For this review, take the finished solid that the model builds, in its own axes (mm). A direction names the side the tool comes from. Coordinates: 2 decimals unless noted, no trailing zeros. Loops run counter-clockwise (first coordinate to the right, second up) from the corner with the lowest first, then second, coordinate; pieces in that order, holes last. Notation, with made-up numbers: (56, -4) -> (101, -4) arc R16 ccw to (101, 20) -> close; hole circle Ø8 at (3.5, -3). An arc over 180 degrees is marked (long way). Answer in a Markdown table with one row per item.
from build123d import *

# Parameters (mm, degrees)
SKETCH1_R                = 2.75
BOSS_EXTRUDE1_DEPTH      = 1
BOSS_EXTRUDE1_DEPTH_BACK = 8.525
CHAMFER1_SIZE            = 10
CHAMFER2_SIZE            = 1
SKETCH2_R                = 1.7
CUT_EXTRUDE1_DEPTH       = 97.192388155
SKETCH3_R                = 1.1
CUT_EXTRUDE2_DEPTH       = 97.192388155
SKETCH4_R                = 3.175
CUT_EXTRUDE3_DEPTH       = 3


with BuildPart() as part:
    # Sketch1 → Boss-Extrude1 (new body, two sides)
    with BuildSketch(Plane.XY) as boss_extrude1_sk:
        Polygon((-1071, 209.41125497), (-1071, 239.41125497), (-1159.192388155, 239.41125497), (-1159.192388155, 259.41125497), (-1167.192388155, 259.41125497), (-1167.192388155, 209.41125497), align=None)
        with Locations((-1122.192388155, 224.41125497)):
            Circle(SKETCH1_R, mode=Mode.SUBTRACT)
        with Locations((-1142.192388155, 224.41125497)):
            Circle(SKETCH1_R, mode=Mode.SUBTRACT)
    extrude(amount=BOSS_EXTRUDE1_DEPTH)
    extrude(boss_extrude1_sk.sketch, amount=-BOSS_EXTRUDE1_DEPTH_BACK)

    # Chamfer1
    chamfer1_edges = [part.edges().sort_by_distance(p)[0] for p in [
        (-1071, 209.41125497, -3.7625),
    ]]
    chamfer(chamfer1_edges, length=CHAMFER1_SIZE)

    # Chamfer2
    chamfer2_edges = [part.edges().sort_by_distance(p)[0] for p in [
        (-1167.192388155, 209.41125497, -3.7625),
        (-1071, 239.41125497, -3.7625),
    ]]
    chamfer(chamfer2_edges, length=CHAMFER2_SIZE)

    # Sketch2 → Cut-Extrude1 (cut, through all)
    with BuildSketch(Plane.ZY.offset(1167.192388155)):
        with Locations((-3.762499999, 249.41125497)):
            Circle(SKETCH2_R)
    extrude(amount=-CUT_EXTRUDE1_DEPTH, mode=Mode.SUBTRACT)

    # Sketch3 → Cut-Extrude2 (cut, through all)
    with BuildSketch(Plane.ZY.offset(1167.192388155)):
        with Locations((-3.762499999, 255.41125497)):
            Circle(SKETCH3_R)
        with Locations((-3.762499999, 243.41125497)):
            Circle(SKETCH3_R)
    extrude(amount=-CUT_EXTRUDE2_DEPTH, mode=Mode.SUBTRACT)

    # Sketch4 → Cut-Extrude3 (cut)
    with BuildSketch(Plane.ZY.offset(1167.192388155)):
        with Locations((-3.762499999, 249.41125497)):
            Circle(SKETCH4_R)
    extrude(amount=-CUT_EXTRUDE3_DEPTH, mode=Mode.SUBTRACT)


solid = part.part
Item 1: Take a section at D-D, the plane x = -1124. State the section outline as (y, z) points (3 decimals), and give its area (3 significant figures).
Worked answers:
| item | result |
|---|---|
| outline | (209.411, -8.525) -> (222.339, -8.525) -> (222.339, 1) -> (209.411, 1) -> close; (226.484, -8.525) -> (239.411, -8.525) -> (239.411, 1) -> (226.484, 1) -> close |
| area | 246 mm² |
Item 2: Take a section at C-C, the plane y = 241. State the section outline as (x, z) points (3 decimals).
Worked answers:
| item | result |
|---|---|
| outline | (-1167.192, -8.525) -> (-1159.192, -8.525) -> (-1159.192, 1) -> (-1167.192, 1) -> close |
Item 3: Take a section at A-A, the plane x = -1142. State the section outline as (y, z) points (3 decimals).
Worked answers:
| item | result |
|---|---|
| outline | (209.411, -8.525) -> (221.668, -8.525) -> (221.668, 1) -> (209.411, 1) -> close; (227.155, -8.525) -> (239.411, -8.525) -> (239.411, 1) -> (227.155, 1) -> close |
Item 4: For faces 4 (the flat face through (-1120, 229, -8.525)), 5 (the flat face through (-1159.192, 249, -6)), 6 (the flat face through (-1164.192, 248, -2)), list the 3-axis set-ups (+Z, -Z, +X, -X, +Y, -Y) from which the entire face can be reached by the end or side of a thin tool; tool diameter is ignored.
Worked answers:
| item | result |
|---|---|
| face 4 | -Z, +X, -X, +Y, -Y |
| face 5 | +Z, -Z, +X, +Y |
| face 6 | -X |
Item 5: The part is to be moulded in two halves that separate along Z. For faces 1 (the cylindrical face through (-1163.248, 242.337, -4.001)), 2 (the flat face through (-1076.07, 214.34, -3.7)), 3 (the flat face through (-1120, 229, 1)), say which applies: +Z half, -Z half, draft (parallel to the pull), parting line (faces both ways), or undercut.
Worked answers:
| item | result |
|---|---|
| face 1 | undercut |
| face 2 | draft |
| face 3 | +Z half |
Item 6: For L1, parallel to X at y = 224.5, z = -4.5; L2, parallel to X at y = 253.5, z = -6.25; L3, parallel to Y at x = -1125, z = 0, list the stretches that pass through material, from the lowest coordinate up.
Worked answers:
| item | result |
|---|---|
| L1 | -1167.19 to -1144.94, -1139.44 to -1124.94, -1119.44 to -1071 |
| L2 | -1167.19 to -1159.19 |
| L3 | 209.41 to 239.41 |
Item 7: Take a section at B-B, the plane x = -1154. State the section outline as (y, z) points (3 decimals).
Worked answers:
| item | result |
|---|---|
| outline | (209.411, -8.525) -> (239.411, -8.525) -> (239.411, 1) -> (209.411, 1) -> close |
Item 8: Insertion check: pin 1 (1.9 mm diameter, centred on y = 250, z = -5, fed in from -X); pin 2 (5 mm diameter, centred on x = -1092.5, z = -6, fed in from +Y); pin 3 (5 mm diameter, centred on y = 252.5, z = -3, fed in from +X). Each pin has a flat end and moves straight along its axis. Give the tip position at first contact, or say it passes through.
Worked answers:
| item | result |
|---|---|
| pin 1 | x = -1164.19 |
| pin 2 | y = 239.41 |
| pin 3 | x = -1159.19 |
